The listing builds one solid part. Answer for the finished solid, in the listing's coordinates (mm). Give positions to 0.01 mm unless a question says otherwise; leave off trailing zeros. Write each loop counter-clockwise with the first axis right and the second up, starting at its lowest first coordinate (ties: lowest second). Pieces come first, ordered by that corner, then holes. Notation, with made-up numbers: M 51.25,85 L 100.25,85 A17 ccw 100.25,93 Z; hole C 26.25,-23.5 d3. An arc over 180 degrees is marked long. Return JSON: item names as keys, results as strings.
from build123d import *

# Parameters (mm, degrees)
F0_R     = 9
F1_DEPTH = 12


with BuildPart() as f1:
    # F0 (on Front) → F1 (new body)
    with BuildSketch(Plane.XZ):
        with BuildLine():
            Line((530, 0), (320, 0))
            Line((320, 0), (320, -785.367647))
            Line((320, -785.367647), (405, -706.617647))
            Line((405, -706.617647), (405, -658.088235))
            ThreePointArc((405, -658.088235), (425, -638.088235), (445, -658.088235))
            Line((445, -658.088235), (445, -706.617647))
            Line((445, -706.617647), (530, -785.367647))
            Line((530, -785.367647), (530, 0))
        make_face()
        with Locations((370, -650)):
            Circle(F0_R, mode=Mode.SUBTRACT)
        with Locations((480, -650)):
            Circle(F0_R, mode=Mode.SUBTRACT)
        with Locations((370, -350)):
            Circle(F0_R, mode=Mode.SUBTRACT)
        with Locations((370, -50)):
            Circle(F0_R, mode=Mode.SUBTRACT)
        with Locations((480, -350)):
            Circle(F0_R, mode=Mode.SUBTRACT)
        with Locations((480, -50)):
            Circle(F0_R, mode=Mode.SUBTRACT)
    extrude(amount=F1_DEPTH)


solid = f1.part
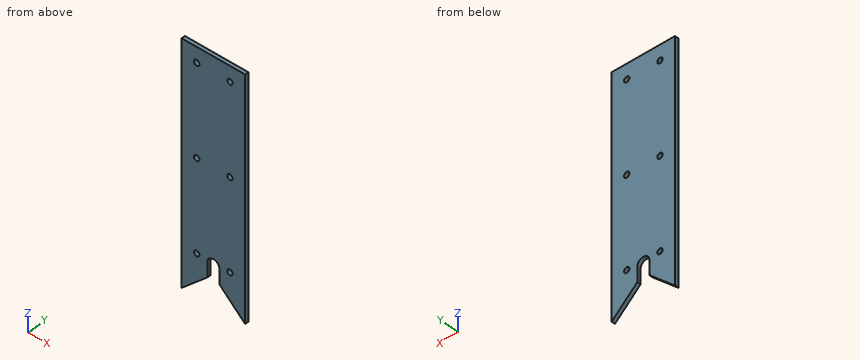
Item 1: Find the intervals of material crossed by line 1 (Z direction, x = 371, y = -2.75); line 2 (Z direction, x = 480, y = -6.5); line 3 (Z direction, x = 411.5, y = -6.5), in increasing order.
Geometry results:
{"line 1": "z = -738.12 to -658.94, -641.06 to -358.94, -341.06 to -58.94, -41.06 to 0", "line 2": "z = -739.04 to -659, -641 to -359, -341 to -59, -41 to 0", "line 3": "z = -643.33 to 0"}
Item 2: A cutting plane is placed at C-C, the plane z = -50. Write down the section's boundary in (x, y), plus the area to 3 significant figures.
Geometry results:
{"outline": "M 320,-12 L 361,-12 L 361,0 L 320,0 Z; M 379,-12 L 471,-12 L 471,0 L 379,0 Z; M 489,-12 L 530,-12 L 530,0 L 489,0 Z", "area": "2,090 mm2"}
Item 3: A cutting plane is placed at A-A, the plane z = -684.5. Write down the section's boundary in (x, y), plus the area to 3 significant figures.
Geometry results:
{"outline": "M 320,-12 L 405,-12 L 405,0 L 320,0 Z; M 445,-12 L 530,-12 L 530,0 L 445,0 Z", "area": "2,040 mm2"}
Item 4: A cutting plane is placed at B-B, the plane y = -2. Write down the section's boundary in (x, z), plus the area to 3 significant figures.
Geometry results:
{"outline": "M 320,-785.37 L 405,-706.62 L 405,-658.09 A20 cw 445,-658.09 L 445,-706.62 L 530,-785.37 L 530,0 L 320,0 Z; hole C 370,-650 d18; hole C 370,-350 d18; hole C 370,-50 d18; hole C 480,-650 d18; hole C 480,-350 d18; hole C 480,-50 d18", "area": "151,000 mm2"}
Item 5: A cutting plane is placed at D-D, the plane x = 370.5. Write down the section's boundary in (y, z), plus the area to 3 significant figures.
Geometry results:
{"outline": "M -12,-738.58 L 0,-738.58 L 0,-658.99 L -12,-658.99 Z; M -12,-641.01 L 0,-641.01 L 0,-358.99 L -12,-358.99 Z; M -12,-341.01 L 0,-341.01 L 0,-58.99 L -12,-58.99 Z; M -12,-41.01 L 0,-41.01 L 0,0 L -12,0 Z", "area": "8,220 mm2"}
Item 6: Given pin 1 Ø1 at (x, y) = (416.5, -6) entering from -Z; pin 2 Ø1.5 at (x, y) = (503, -8.5) entering from -Z, each flat-ended and moving along its own axis, determine where each tip first touches the part or whether it passes through.
Geometry results:
{"pin 1": "stops at z = -640.23", "pin 2": "stops at z = -761.05"}
